Can you work these out from the model? Positions are in its coordinate system, mm. Face numbers are marked on the shaded views. Coordinates: 2 decimals unless noted, no trailing zeros. Write each loop counter-clockwise with the first axis right and the second up, starting at its lowest first coordinate (ties: lowest second). Pieces come first, ordered by that corner, then holes.
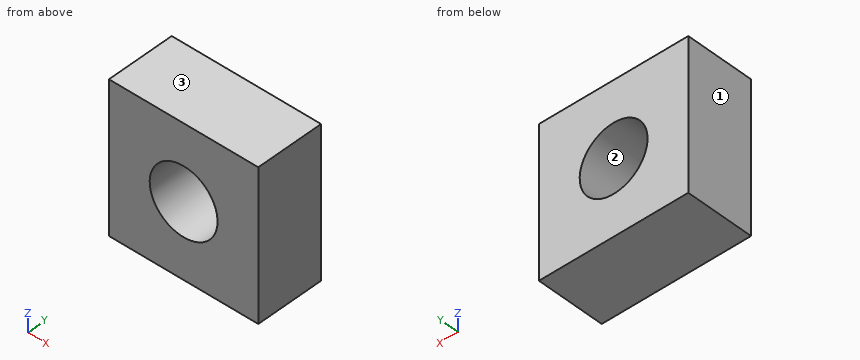
```python
from build123d import *

# Parameters (mm, degrees)
SKETCH1_W           = 5.5
SKETCH1_H           = 5.5
BOSS_EXTRUDE1_DEPTH = 1.25
SKETCH4_W           = 1.25
SKETCH4_H           = 2.501


with BuildPart() as part:
    # Sketch1 → Boss-Extrude1 (new body, symmetric)
    with BuildSketch(Plane(origin=(0, 0, 0), x_dir=(1, 0, 0), z_dir=(0, 1, 0))):
        Rectangle(SKETCH1_W, SKETCH1_H)
    extrude(amount=BOSS_EXTRUDE1_DEPTH, both=True)

    # Sketch4 → Tap Drill for M3x0.5 Tap1 (revolve, cut)
    with BuildSketch(Plane(origin=(0, 1.25, 0), x_dir=(0, 0, 1), z_dir=(1, 0, 0))):
        with Locations((0.625, 1.2505)):
            Rectangle(SKETCH4_W, SKETCH4_H)
    revolve(axis=Axis((0, 7.6, 0), (0, -1, 0)), mode=Mode.SUBTRACT)


solid = part.part
```
1. If I drill on L1, parallel to Z at x = 0, y = 0.15; L2, parallel to Z at x = 0.75, y = -0.7, over which ranges is the centre line in solid material (lowest first)?
2. I'm going to push a flat-ended pin straight in: P1, Ø1.5, axis at x = 0, z = 0, coming from the -Y side. Where does the tip first touch, or does it pass through?
3. If we section it at A-A, the plane x = 1.1: List the corners of the cut face in (y, z) for me.
4. If we section it at B-B, the plane z = 0: List the corners of the cut face in (x, y) for me, plus the area to 3 significant figures.
5. We'd pull the mould along Z, two halves only. Please class the marked faces 1, 2 and 3: released by +Z, released by -Z, zero draft, split by the parting line, or undercut.
6. If we section it at C-C, the plane y = 0.6: List the corners of the cut face in (x, z) for me.
Answers:
1. L1: z = -2.75 to -1.25, 1.25 to 2.75
1. L2: z = -2.75 to -1, 1 to 2.75
2. P1: passes through
3. outline: (-1.25, -2.75) - (1.25, -2.75) - (1.25, -0.59) - (-1.25, -0.59) - close; (-1.25, 0.59) - (1.25, 0.59) - (1.25, 2.75) - (-1.25, 2.75) - close
4. outline: (-2.75, -1.25) - (-1.25, -1.25) - (-1.25, 1.25) - (-2.75, 1.25) - close; (1.25, -1.25) - (2.75, -1.25) - (2.75, 1.25) - (1.25, 1.25) - close
4. area: 7.50 mm2
5. face 1: zero draft
5. face 2: undercut
5. face 3: released by +Z
6. outline: (-2.75, -2.75) - (2.75, -2.75) - (2.75, 2.75) - (-2.75, 2.75) - close; hole circle Ø2.5 at (0, 0)
